Source: CAD feature listing. Evaluate the final solid. Frame: model axes, mm. Face numbers are marked on the shaded views. Coordinates: 2 decimals unless noted, no trailing zeros. Order: outer loops, then holes, each group sorted by start corner. A loop starts at its lowest first (then second) coordinate and runs counter-clockwise, first axis right, second up. Notation, with made-up numbers: (-39, 87) - (-4, 87) arc R14 cw to (-4, 113) - close; hole circle Ø3 at (-33.75, -17.75). An arc over 180 degrees is marked (long way). One line per question, with ' | ' between items. Start each with the question number.
(1) Section B-B (y = -18). Return the cut outline in (x, z).
(2) Section C-C (x = 107.5). Return the cut outline in (y, z), then the cut area to 3 significant figures.
(3) Draft query along Z for the marked faces 1, 2, 3 and 4. Return one class per face: +Z half, -Z half, draft (parallel to the pull), parting line (faces both ways), or undercut.
(4) Contact query for flat-ended pins moving along their axis: P1, Ø2, axis at x = 26, z = -6.5, coming from the +Y side; P2, Ø2, axis at x = 10.5, z = -67, coming from the -Y side. Output: stop coordinate, or through.
(5) Section A-A (x = 54). Return the cut outline in (y, z), then the cut area to 3 significant figures.
(6) Line query: line 1 along Z through (x, y) = (87, -22); line 2 along Y through (x, z) = (99, -65.5). Output: solid intervals per line, ascending.
from build123d import *

# Parameters (mm, degrees)
BOSS_EXTRUDE1_DEPTH = 7.62
SKETCH5_W           = 158.75
SKETCH5_H           = 12.7
BOSS_EXTRUDE2_DEPTH = 25.4
FILLET1_R           = 5.08
SKETCH3_R           = 1.397
SKETCH3_R_2         = 1.524
CUT_EXTRUDE1_DEPTH  = 7.62
SKETCH6_W           = 7.62
SKETCH6_H           = 2.54
CUT_EXTRUDE3_DEPTH  = 7.62


with BuildPart() as part:
    # Sketch1 → Boss-Extrude1 (new body)
    with BuildSketch(Plane(origin=(0, 0, 0), x_dir=(1, 0, 0), z_dir=(0, 1, 0))):
        Polygon((0, 0), (120.65, 0), (120.65, 142.24), (-38.1, 142.24), (-38.1, 0), align=None)
    extrude(amount=BOSS_EXTRUDE1_DEPTH)

    # Sketch5 → Boss-Extrude2 (add)
    with BuildSketch(Plane(origin=(0, 0, 0), x_dir=(-1, 0, 0), z_dir=(0, -1, 0))):
        with Locations((-41.275, 6.35)):
            Rectangle(SKETCH5_W, SKETCH5_H)
        with Locations((-41.275, 135.89)):
            Rectangle(SKETCH5_W, SKETCH5_H)
    extrude(amount=BOSS_EXTRUDE2_DEPTH)

    # Fillet1
    fillet1_edges = [part.edges().sort_by_distance(p)[0] for p in [
        (-38.1, -8.89, 0),
        (-38.1, -8.89, -142.24),
        (120.65, -8.89, -142.24),
        (120.65, -8.89, 0),
    ]]
    fillet(fillet1_edges, radius=FILLET1_R)

    # Sketch3 → Cut-Extrude1 (cut)
    with BuildSketch(Plane(origin=(0, 7.62, 0), x_dir=(1, 0, 0), z_dir=(0, 1, 0))):
        with Locations(Location((25.781, 6.731, 0), (0, 0, 270))):
            Circle(SKETCH3_R)
        with Locations(Location((25.781, 55.4355, 0), (0, 0, 270))):
            Circle(SKETCH3_R)
        with Locations(Location((84.455, 55.499, 0), (0, 0, 270))):
            Circle(SKETCH3_R)
        with Locations(Location((84.455, 6.731, 0), (0, 0, 270))):
            Circle(SKETCH3_R)
        with Locations(Location((-34.036, 137.16, 0), (0, 0, 270))):
            Circle(SKETCH3_R_2)
        with Locations(Location((0, 137.16, 0), (0, 0, 270))):
            Circle(SKETCH3_R_2)
        with Locations(Location((-34.036, 113.284, 0), (0, 0, 270))):
            Circle(SKETCH3_R_2)
        with Locations(Location((0, 113.284, 0), (0, 0, 270))):
            Circle(SKETCH3_R_2)
        with Locations(Location((-34.036, 103.632, 0), (0, 0, 270))):
            Circle(SKETCH3_R_2)
        with Locations(Location((0, 103.632, 0), (0, 0, 270))):
            Circle(SKETCH3_R_2)
        with Locations(Location((-34.036, 79.756, 0), (0, 0, 270))):
            Circle(SKETCH3_R_2)
        with Locations(Location((0, 79.756, 0), (0, 0, 270))):
            Circle(SKETCH3_R_2)
        with Locations(Location((-34.036, 70.104, 0), (0, 0, 270))):
            Circle(SKETCH3_R_2)
        with Locations(Location((0, 70.104, 0), (0, 0, 270))):
            Circle(SKETCH3_R_2)
        with Locations(Location((-34.036, 46.228, 0), (0, 0, 270))):
            Circle(SKETCH3_R_2)
        with Locations(Location((0, 46.228, 0), (0, 0, 270))):
            Circle(SKETCH3_R_2)
        with Locations(Location((-27.178, 14.003291804, 0), (0, 0, 270))):
            Circle(SKETCH3_R_2)
        with Locations(Location((-27.269651582, 29.334943362, 0), (0, 0, 270))):
            Circle(SKETCH3_R_2)
    extrude(amount=-CUT_EXTRUDE1_DEPTH, mode=Mode.SUBTRACT)

    # Sketch6 → Cut-Extrude3 (cut)
    with BuildSketch(Plane(origin=(0, 7.62, 0), x_dir=(1, 0, 0), z_dir=(0, 1, 0))):
        with Locations((55.167188758, 70.832515898)):
            Rectangle(SKETCH6_W, SKETCH6_H)
        with Locations((55.167188758, 98.772515898)):
            Rectangle(SKETCH6_W, SKETCH6_H)
    extrude(amount=-CUT_EXTRUDE3_DEPTH, mode=Mode.SUBTRACT)


solid = part.part
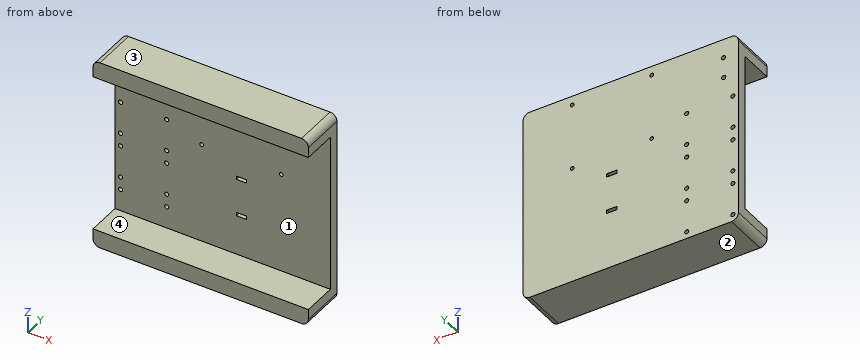
Response values:
1) outline: (-38.1, -137.16) arc R5.08 ccw to (-33.02, -142.24) - (115.57, -142.24) arc R5.08 ccw to (120.65, -137.16) - (120.65, -129.54) - (-38.1, -129.54) - close; (-38.1, -12.7) - (120.65, -12.7) - (120.65, -5.08) arc R5.08 ccw to (115.57, 0) - (-33.02, 0) arc R5.08 ccw to (-38.1, -5.08) - close
2) outline: (-25.4, -142.24) - (7.62, -142.24) - (7.62, 0) - (-25.4, 0) - (-25.4, -12.7) - (0, -12.7) - (0, -129.54) - (-25.4, -129.54) - close | area: 1,730 mm²
3) face 1: undercut | face 2: -Z half | face 3: +Z half | face 4: undercut
4) P1: stops at y = 0 | P2: stops at y = 0
5) outline: (-25.4, -142.24) - (7.62, -142.24) - (7.62, -100.04) - (0, -100.04) - (0, -129.54) - (-25.4, -129.54) - close; (-25.4, -12.7) - (0, -12.7) - (0, -69.56) - (7.62, -69.56) - (7.62, 0) - (-25.4, 0) - close; (0, -97.5) - (7.62, -97.5) - (7.62, -72.1) - (0, -72.1) - close | area: 1,690 mm²
6) line 1: z = -142.24 to -129.54, -12.7 to 0 | line 2: y = 0 to 7.62
